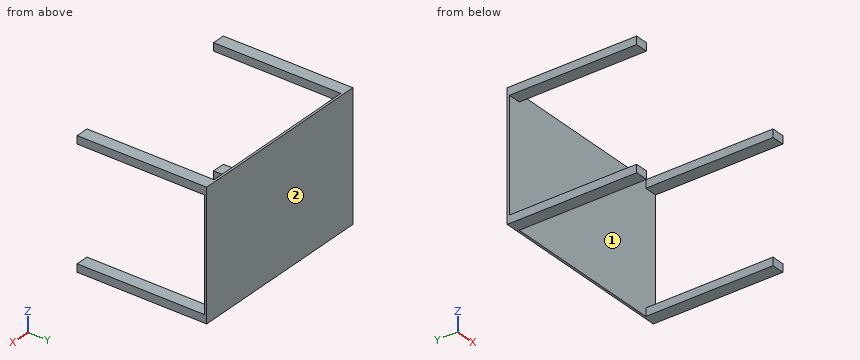
```python
from build123d import *

# Parameters (mm, degrees)
F0_W     = 600
F0_H     = 400
F1_DEPTH = 7
F2_W     = 40
F2_H     = 25
F3_DEPTH = 400
F4_DEPTH = 400
F5_DEPTH = 400
F6_DEPTH = 400


with BuildPart() as f1:
    # F0 (on Front) → F1 (new body)
    with BuildSketch(Plane.XZ):
        with Locations((93.126289, 59.305324)):
            Rectangle(F0_W, F0_H)
    extrude(amount=F1_DEPTH)

    # F2 (on face) → F3 (join)
    with BuildSketch(Plane.XZ.offset(7)):
        with Locations((-186.873711, 246.805324)):
            Rectangle(F2_W, F2_H)
    extrude(amount=F3_DEPTH)

    # F2 (on face) → F4 (join)
    with BuildSketch(Plane.XZ.offset(7)):
        with Locations((-186.873711, -128.194676)):
            Rectangle(F2_W, F2_H)
    extrude(amount=F4_DEPTH)

    # F2 (on face) → F5 (join)
    with BuildSketch(Plane.XZ.offset(7)):
        with Locations((373.126289, 246.805324)):
            Rectangle(F2_W, F2_H)
    extrude(amount=F5_DEPTH)

    # F2 (on face) → F6 (join)
    with BuildSketch(Plane.XZ.offset(7)):
        with Locations((373.126289, -128.194676)):
            Rectangle(F2_W, F2_H)
    extrude(amount=F6_DEPTH)


solid = f1.part
```
Verification items for the finished model (mm, model axes). Face numbers are marked on the shaded views. Round coordinates to 2 decimals unless told otherwise and drop trailing zeros. Loops run counter-clockwise (first coordinate to the right, second up) from the corner with the lowest first, then second, coordinate; pieces in that order, holes last. Notation, with made-up numbers: (45.25, 18.5) -> (49.25, 18.5) arc R29 cw to (49.25, 48.5) -> close; hole circle Ø1 at (-16.75, -33). An arc over 180 degrees is marked (long way). Answer as a JSON object with one key per item and string values.
Q1. Go/stop test with a flat-tipped pin: P1, Ø2, axis at x = 50, z = 191.5, coming from the +Y side. Record where the tip stops, or that it passes through.
Data:
{"P1": "stops at y = 0"}
Q2. Section check A-A (y = -272). Record the boundary of the cut face in (x, z).
Data:
{"outline": "(-206.87, -140.69) -> (-166.87, -140.69) -> (-166.87, -115.69) -> (-206.87, -115.69) -> close; (-206.87, 234.31) -> (-166.87, 234.31) -> (-166.87, 259.31) -> (-206.87, 259.31) -> close; (353.13, -140.69) -> (393.13, -140.69) -> (393.13, -115.69) -> (353.13, -115.69) -> close; (353.13, 234.31) -> (393.13, 234.31) -> (393.13, 259.31) -> (353.13, 259.31) -> close"}
Q3. Scan lines: line 1 (X direction, y = -193.5, z = 238); line 2 (Y direction, x = 106, z = 91.5). Record each from-to range of solid material in increasing order. Write a range as from..to.
Data:
{"line 1": "x = -206.87..-166.87, 353.13..393.13", "line 2": "y = -7..0"}
Q4. Section check B-B (z = 107). Record the boundary of the cut face in (x, y), then the cut area to 3 significant figures.
Data:
{"outline": "(-206.87, -7) -> (393.13, -7) -> (393.13, 0) -> (-206.87, 0) -> close", "area": "4,200 mm2"}
Q5. Draft check along Z on the marked faces 1 and 2. Enter one of: pulls with the +Z half, pulls with the -Z half, needs draft (parallel to the pull), parting line crosses it, or undercut.
Data:
{"face 1": "undercut", "face 2": "needs draft"}
Q6. Section check C-C (x = 194). Record the boundary of the cut face in (y, z).
Data:
{"outline": "(-7, -140.69) -> (0, -140.69) -> (0, 259.31) -> (-7, 259.31) -> close"}
